Model file for the job. Use its own axes, mm. A direction names the side the tool comes from. Round coordinates to 2 decimals unless told otherwise and drop trailing zeros. Loops run counter-clockwise (first coordinate to the right, second up) from the corner with the lowest first, then second, coordinate; pieces in that order, holes last. Notation, with made-up numbers: (87, -33.5) -> (99, -33.5) arc R30 cw to (99, 3.5) -> close; hole circle Ø9 at (88, 47.5). An arc over 180 degrees is marked (long way). Use a Markdown table: item, result. Add a question column.
Autodesk Inventor part; units mm, degrees
ref_plane "YZ Plane" through (0, 0, 0) normal (1, 0, 0) x (0, 1, 0)
ref_plane "XZ Plane" through (0, 0, 0) normal (0, 1, 0) x (-1, 0, 0)
ref_plane "XY Plane" through (0, 0, 0) normal (0, 0, 1) x (1, 0, 0)
sketch "Sketch1" plane through (0, 0, 0) normal (0, 0, 1) x (1, 0, 0)
  line L0 (2, 0) -> (2, -17.9997)
  line L1 (226, 217) -> (226, -317)
  arc A0 (226, 0) -> (2, 0) centre (114, 0) ccw
  line L2 (2, -17.9997) -> (5, -17.9997)
  line L3 (5, -17.9997) -> (17, -5.9997)
  line L4 (17, -5.9997) -> (17, 0)
  line L5 (211, 0) -> (211, -275)
  line L6 (211, -275) -> (223, -287)
  line L7 (223, -287) -> (226, -287)
  arc A1 (211, 0) -> (17, 0) centre (114, 0) ccw
  point P0 (0, 0)
  point P1 (114, 112)
  point P2 (114, 97)
  dimension "d0" = 15
  dimension "d1" = 45
  dimension "d2" = 3
  dimension "d3" = 15
  dimension "d4" = 45
  dimension "d5" = 30
  dimension "d6" = 15
extrude "Extrusion1" add sketch "Sketch1" against normal blind 22
equation "\"d3\" = d0"
equation "\"d4\" = d1"
properties part number "Drag Chain Dummy" material "ABS Plastic"
1) Pin check, flat tips, straight feed: pin 1 Ø2 at (y, z) = (25, -9.5) entering from -X; pin 2 Ø1.5 at (x, z) = (159.5, -2.5) entering from +Y; pin 3 Ø6 at (x, z) = (143.5, -17.5) entering from +Y. Stop position of each tip, or through.
2) Pull direction X, two halves, no side cores. Call faces 1 (the face through (116.133, 96.977, -10.846)), 2 (the face through (116.463, 111.973, -10.846)), 3 (the face through (226, -141, -11)): +X half, -X half, draft (parallel to the pull), parting line (faces both ways), or undercut.
3) Wall check: probe 1 along X at (y, z) = (-183.5, -5.5); probe 2 along X at (y, z) = (67, -7); probe 3 along X at (y, z) = (49.5, -5.5). Give the ranges that are in metal, low to high. Write a range as from..to.
4) Tool access for faces 4 (the face through (213, -42, -22)), 5 (the face through (11, -12, -11)): list every direction of +Z, -Z, +X, -X, +Y, -Y with a clear straight run to the whole face (end or side of a thin tool).
5) Cut at A-A on z = -12. Write the cut outline in (x, y), and give its area (3 significant figures).
6) Cut at B-B on y = 26. Write the cut outline in (x, z).
7) Cut at D-D on y = -212.5. Write the cut outline in (x, z), and give its area (3 significant figures).
8) Cut at C-C on x = 114. Write the cut outline in (y, z), and give its area (3 significant figures).
Established:
| question | item | result |
|---|---|---|
| 1 | pin 1 | stops at x = 4.6 |
| 1 | pin 2 | stops at y = 102.67 |
| 1 | pin 3 | stops at y = 108.82 |
| 2 | face 1 | undercut |
| 2 | face 2 | parting line |
| 2 | face 3 | +X half |
| 3 | probe 1 | x = 211..226 |
| 3 | probe 2 | x = 24.25..43.86, 184.14..203.75 |
| 3 | probe 3 | x = 13.53..30.58, 197.42..214.47 |
| 4 | face 4 | -Z, +X, -X, +Y, -Y |
| 4 | face 5 | +Z, -Z, -Y |
| 5 | outline | (2, -18) -> (5, -18) -> (17, -6) -> (17, 0) arc R97 cw to (211, 0) -> (211, -275) -> (223, -287) -> (226, -287) -> (226, 0) arc R112 ccw to (2, 0) -> close |
| 5 | area | 9,360 mm^2 |
| 6 | outline | (5.06, -22) -> (20.55, -22) -> (20.55, 0) -> (5.06, 0) -> close; (207.45, -22) -> (222.94, -22) -> (222.94, 0) -> (207.45, 0) -> close |
| 7 | outline | (211, -22) -> (226, -22) -> (226, 0) -> (211, 0) -> close |
| 7 | area | 330 mm^2 |
| 8 | outline | (97, -22) -> (112, -22) -> (112, 0) -> (97, 0) -> close |
| 8 | area | 330 mm^2 |
